```python
from build123d import *

# Parameters (mm, degrees)
SKETCH1_R           = 3
BOSS_EXTRUDE1_DEPTH = 2


with BuildPart() as part:
    # Sketch1 → Boss-Extrude1 (new body)
    with BuildSketch(Plane(origin=(0, 0, 0), x_dir=(1, 0, 0), z_dir=(0, 1, 0))):
        with BuildLine():
            add(Edge.make_bspline(
                [(-2.75743509, -2.75743509), (0, -17.770137247), (2.75743509, -2.75743509)],
                knots=[1.975688113, 1.975688113, 1.975688113, 4.307497194, 4.307497194, 4.307497194], degree=2, weights=[1, 0.393919299, 1]))
            add(Edge.make_bspline(
                [(2.75743509, -2.75743509), (17.770137247, 0), (2.75743509, 2.75743509)],
                knots=[5.117280767, 5.117280767, 5.117280767, 7.449089848, 7.449089848, 7.449089848], degree=2, weights=[1, 0.393919299, 1]))
            add(Edge.make_bspline(
                [(2.75743509, 2.75743509), (0, 17.770137247), (-2.75743509, 2.75743509)],
                knots=[5.117280767, 5.117280767, 5.117280767, 7.449089848, 7.449089848, 7.449089848], degree=2, weights=[1, 0.393919299, 1]))
            add(Edge.make_bspline(
                [(-2.75743509, 2.75743509), (-17.770137247, 0), (-2.75743509, -2.75743509)],
                knots=[1.975688113, 1.975688113, 1.975688113, 4.307497194, 4.307497194, 4.307497194], degree=2, weights=[1, 0.393919299, 1]))
        make_face()
        Circle(SKETCH1_R, mode=Mode.SUBTRACT)
    extrude(amount=BOSS_EXTRUDE1_DEPTH)


solid = part.part
```
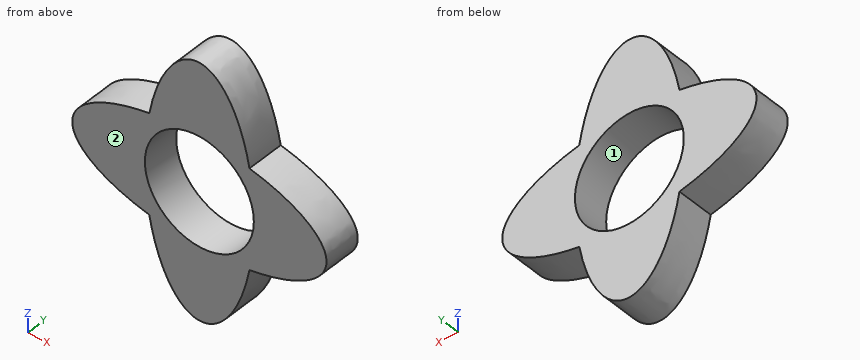
The listing builds one solid part. Answer for the finished solid, in the listing's coordinates (mm). Face numbers are marked on the shaded views. Give positions to 0.01 mm unless a question says otherwise; leave off trailing zeros. Answer as CSV lines item,"result". Start each with the question number.
Item 1: Find the intervals of material crossed by line 1 (Z direction, x = 0, y = 0.8); line 2 (Z direction, x = 1.75, y = 0.1), in increasing order. Write a range as from..to.
Item 2: This flat-tipped pin is pushed along its axis until it touches: pin 1 (4 mm diameter, centred on x = 3, z = -3.5, fed in from +Y). Where does it stop, or does it pass through?
Item 3: The mould has two halves that part along X. Classify the marked faces 1 and 2: +X half, -X half, draft (parallel to the pull), parting line (faces both ways), or undercut.
Found:
1,line 1,"z = -7..-3, 3..7"
1,line 2,"z = -5.69..-2.44, 2.44..5.69"
2,pin 1,"stops at y = 2"
3,face 1,"undercut"
3,face 2,"draft"
